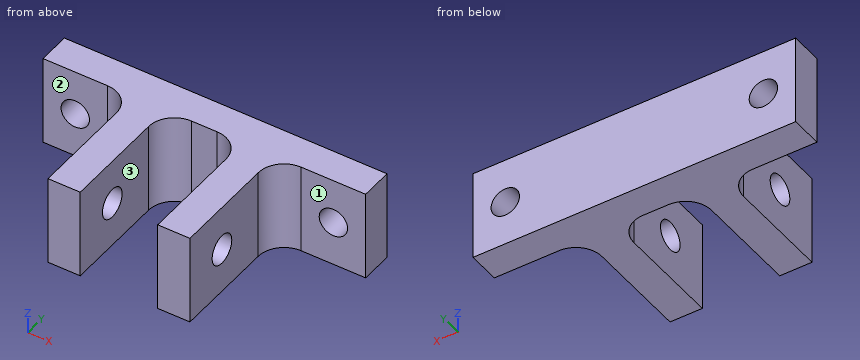
from build123d import *

# Parameters (mm, degrees)
PAD_DEPTH       = 14
SKETCH001_R     = 2.3
POCKET_DEPTH    = 36.001
SKETCH002_R     = 2.2
POCKET001_DEPTH = 25.001
FILLET_R        = 4


with BuildPart() as part:
    # Sketch → Pad (new body)
    with BuildSketch(Plane.XY):
        Polygon((27.992845, 15.579944), (-22.007155, 15.579944), (-22.007155, 10.579944), (-8.007155, 10.579944), (-8.007155, -9.420056), (-3.007155, -9.420056), (-3.007155, 10.579944), (8.992845, 10.579944), (8.992845, -9.420056), (13.992845, -9.420056), (13.992845, 10.579944), (27.992845, 10.579944), align=None)
    extrude(amount=PAD_DEPTH)

    # Sketch001 → Pocket (cut, through all)
    with BuildSketch(Plane.YZ.offset(13.992845)):
        with Locations((-1.920056, 7)):
            Circle(SKETCH001_R)
    extrude(amount=-POCKET_DEPTH, mode=Mode.SUBTRACT)

    # Sketch002 → Pocket001 (cut, through all)
    with BuildSketch(Plane(origin=(0, 15.579944, 0), x_dir=(-1, 0, 0), z_dir=(0, 1, 0))):
        with Locations((-22.992845, 7)):
            Circle(SKETCH002_R)
        with Locations((17.007155, 7)):
            Circle(SKETCH002_R)
    extrude(amount=-POCKET001_DEPTH, mode=Mode.SUBTRACT)

    # Fillet
    fillet_edges = [part.edges().sort_by_distance(p)[0] for p in [
        (13.992845, 10.579944, 7),
        (-8.007155, 10.579944, 7),
        (8.992845, 10.579944, 7),
        (-3.007155, 10.579944, 7),
    ]]
    fillet(fillet_edges, radius=FILLET_R)


solid = part.part
Can you work these out from the model? Positions are in its coordinate system, mm. Face numbers are marked on the shaded views. A direction names the side the tool comes from. Round coordinates to 2 decimals unless told otherwise and drop trailing zeros. Write each loop counter-clockwise with the first axis right and the second up, starting at its lowest first coordinate (ties: lowest second). Pieces come first, ordered by that corner, then holes. Notation, with made-up numbers: (54, 39.25) -> (79, 39.25) arc R32 cw to (79, 68.25) -> close; hole circle Ø5 at (72, 78.5). An arc over 180 degrees is marked (long way). Use one line per item in the form item = value. Start each with the question number.
Q1. Imagine slicing it at C-C (z = 3.75). Please give me the cut outline in (x, y).
Q2. Imagine slicing it at D-D (x = -5). Please give me the cut outline in (y, z), then the cut area to 3 significant figures.
Q3. If I drill on probe 1 along X at (y, z) = (-6.75, 3.25); probe 2 along Y at (x, z) = (20.5, 8); probe 3 along X at (y, z) = (9.75, 12), over which ranges is the centre line in solid material (lowest first)? Write a range as [from, to].
Q4. Imagine slicing it at A-A (y = 4.75). Please give me the cut outline in (x, z).
Q5. Imagine slicing it at B-B (z = 7). Count the separate pieces of the cut face and the enclosed holes in it, then the cut area to 3 significant figures.
Q6. I'm going to push flat-ended pins straight in: P1, Ø1.2, axis at x = 2.5, z = 9, coming from the -Y side; P2, Ø4, axis at y = -5, z = 7, coming from the +X side; P3, Ø6, axis at y = -1.92, z = 7, coming from the -X side; P4, Ø3.5, axis at x = -17.01, z = 7, coming from the +Y side. Where does each tip first touch, or does it pass through?
Q7. Which directions (+Z, -Z, +X, -X, +Y, -Y) give clear straight access to the entire face, cutting with the end or side of a thin tool? Please do the marked faces 1, 2 and 3.
Worked out:
q1.outline = (-22.01, 10.58) -> (-12.01, 10.58) arc R4 cw to (-8.01, 6.58) -> (-8.01, -9.42) -> (-3.01, -9.42) -> (-3.01, 6.58) arc R4 cw to (0.99, 10.58) -> (4.99, 10.58) arc R4 cw to (8.99, 6.58) -> (8.99, -9.42) -> (13.99, -9.42) -> (13.99, 6.58) arc R4 cw to (17.99, 10.58) -> (27.99, 10.58) -> (27.99, 15.58) -> (-22.01, 15.58) -> close
q2.outline = (-9.42, 0) -> (15.58, 0) -> (15.58, 14) -> (-9.42, 14) -> close; hole circle Ø4.6 at (-1.92, 7)
q2.area = 333 mm^2
q3.probe_1 = [-8.01, -3.01], [8.99, 13.99]
q3.probe_2 = [10.58, 15.58]
q3.probe_3 = [-9.57, -1.45], [7.43, 15.55]
q4.outline = (-8.01, 0) -> (-3.01, 0) -> (-3.01, 14) -> (-8.01, 14) -> close; (8.99, 0) -> (13.99, 0) -> (13.99, 14) -> (8.99, 14) -> close
q5.separate_pieces = 5
q5.enclosed_holes = 0
q5.area = 374 mm^2
q6.P1 = 10.58
q6.P2 = 13.99
q6.P3 = -8.01
q6.P4 = through
q7.face_1 = +Z, -Z, +X, -Y
q7.face_2 = +Z, -Z, -X, -Y
q7.face_3 = +Z, -Z, -Y
